Part print with two shaded views. Sizes in mm from the minimum x, y, z corner. A direction names the side the tool comes from. Coordinates: 2 decimals unless noted, no trailing zeros. Loops run counter-clockwise (first coordinate to the right, second up) from the corner with the lowest first, then second, coordinate; pieces in that order, holes last. Notation, with made-up numbers: (71.5, 9) -> (91.5, 9) arc R21 cw to (91.5, 25) -> close; hole circle Ø7 at (-30.5, 18). An arc over 180 degrees is marked (long way). Return JSON: item names as keys, results as strings. Group by question number.
(1) Tool access for the marked faces 1, 2, 3, 4 and 5: list every direction of +Z, -Z, +X, -X, +Y, -Y with a clear straight run to the whole face (end or side of a thin tool).
(2) Flat gauge pins, fed straight in: pin 1 Ø2.5 at (y, z) = (33.5, 13) entering from -X; pin 2 Ø8 at (x, z) = (51, 15) entering from -Y; pin 3 Ø15 at (x, z) = (36.5, 8.5) entering from -Y. Where does each tip first touch, or does it go through?
(3) Probe L1, parallel to Z at x = 54, y = 5; L2, parallel to Y at x = 11, z = 24.5; L3, parallel to X at y = 17, z = 11. List the from-to ranges inside material, lowest first.
(4) Saw through at C-C on x = 54. Write the cut outline in (y, z), then the cut area to 3 significant figures.
(5) Saw through at A-A on y = 7. Write the cut outline in (x, z), then the cut area to 3 significant figures.
(6) Saw through at D-D on y = 22. Write the cut outline in (x, z).
(7) Saw through at B-B on z = 34. Write the cut outline in (x, y), then the cut area to 3 significant figures.
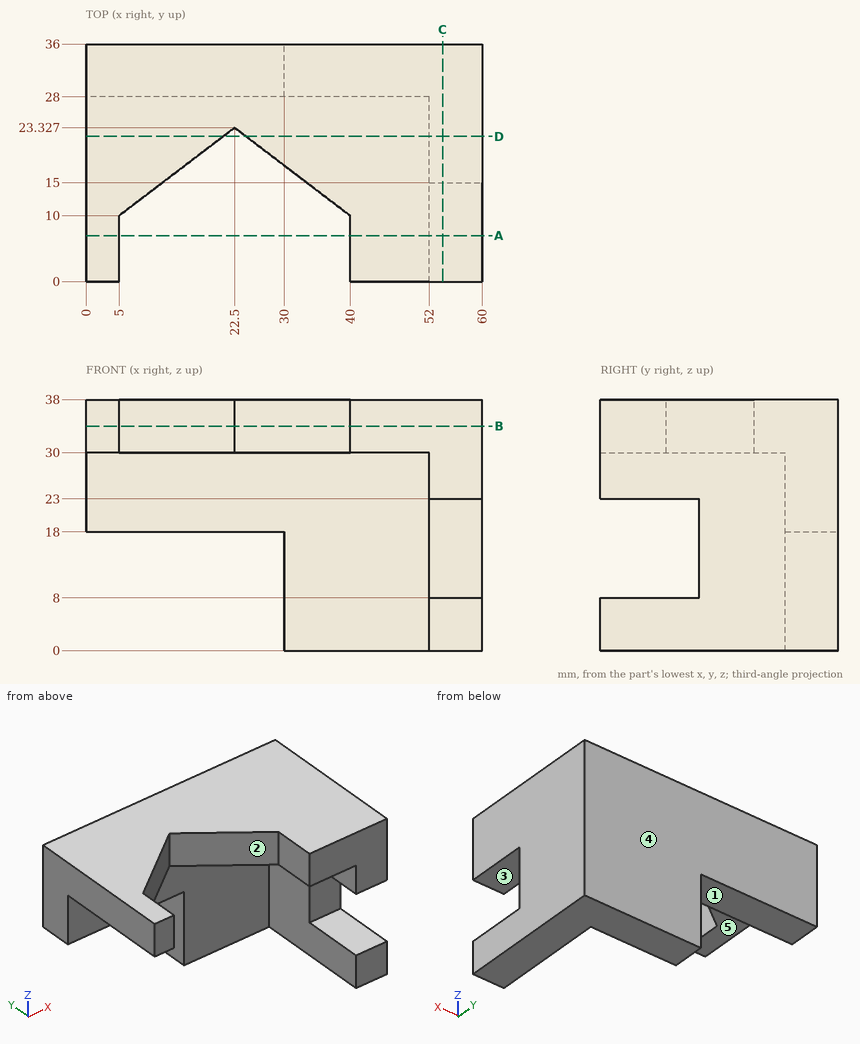
Geometry results:
{
 "1": {"face 1": "-Z, -X, +Y, -Y", "face 2": "+Z, -Z, -Y", "face 3": "+X, -X, -Y", "face 4": "+Z, -Z, +X, -X, +Y", "face 5": "-Z, -X, -Y"},
 "2": {"pin 1": "x = 30", "pin 2": "y = 15", "pin 3": "y = 28"},
 "3": {"L1": "0 to 8, 23 to 38", "L2": "28 to 36", "L3": "52 to 60"},
 "4": {"outline": "(0, 0) -> (36, 0) -> (36, 38) -> (0, 38) -> (0, 23) -> (15, 23) -> (15, 8) -> (0, 8) -> close", "area": "1,140 mm²"},
 "5": {"outline": "(0, 30) -> (5, 30) -> (5, 38) -> (0, 38) -> close; (40, 30) -> (52, 30) -> (52, 23) -> (60, 23) -> (60, 38) -> (40, 38) -> close; (52, 0) -> (60, 0) -> (60, 8) -> (52, 8) -> close", "area": "320 mm²"},
 "6": {"outline": "(0, 30) -> (20.76, 30) -> (20.76, 38) -> (0, 38) -> close; (24.24, 30) -> (52, 30) -> (52, 0) -> (60, 0) -> (60, 38) -> (24.24, 38) -> close"},
 "7": {"outline": "(0, 0) -> (5, 0) -> (5, 10) -> (22.5, 23.33) -> (40, 10) -> (40, 0) -> (60, 0) -> (60, 36) -> (0, 36) -> close", "area": "1,580 mm²"}
}
